The figure shows three views and two pictorial views of one solid part (mm, origin at its lowest corner). Answer the questions. A direction names the side the tool comes from. Coordinates: 2 decimals unless noted, no trailing zeros. Order: outer loops, then holes, each group sorted by start corner. A loop starts at its lowest first (then second) coordinate and runs counter-clockwise, first axis right, second up. Notation, with made-up numbers: (-15, 16) -> (29, 16) arc R16 ccw to (29, 46) -> close; hole circle Ø1 at (-6, 18.5). An arc over 180 degrees is marked (long way). Write item = value, one per line.
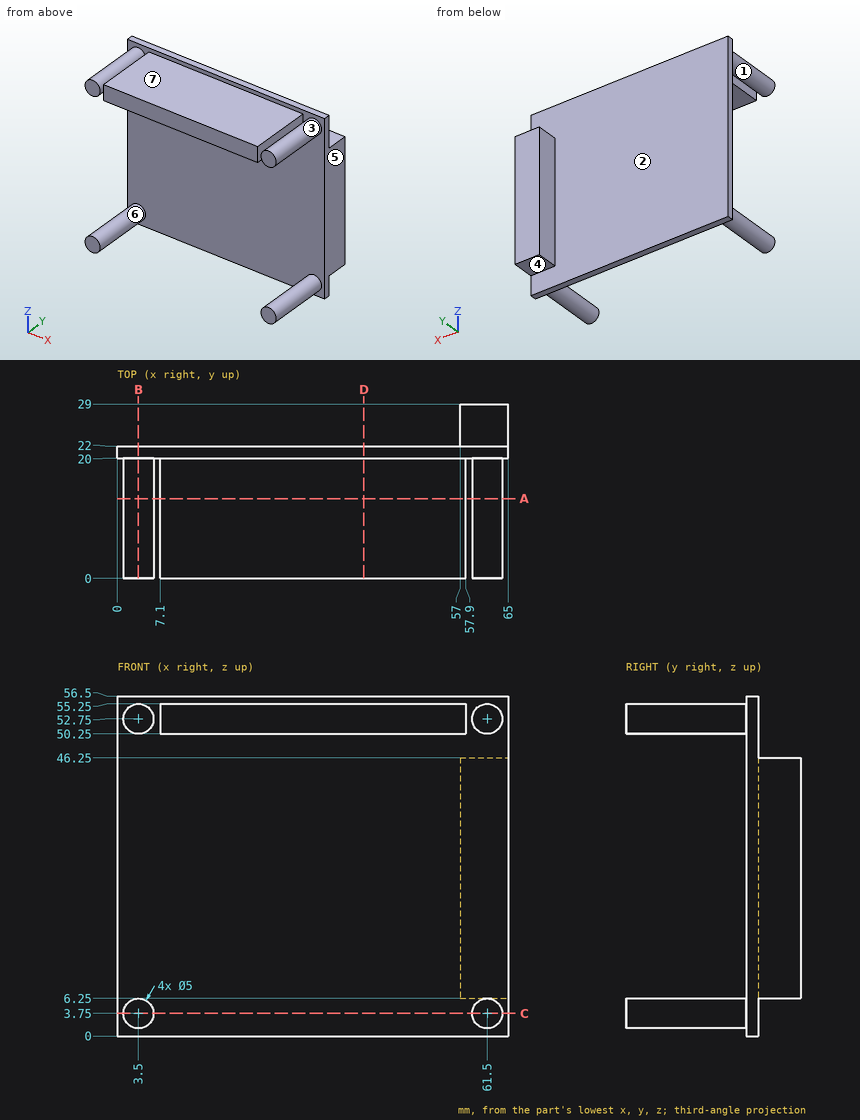
Q1. Find the intervals of material crossed by line 1 along X through (y, z) = (7, 50.5); line 2 along Z through (x, y) = (19.5, 7); line 3 along X through (y, z) = (26.75, 8.5), in increasing order.
The answers:
line_1 = 2.41 to 4.59, 7.1 to 57.9, 60.41 to 62.59
line_2 = 50.25 to 55.25
line_3 = 57 to 65
Q2. The mould has two halves that part along Z. Classify the marked faces 1, 2, 3 and 4: released by +Z, released by -Z, zero draft, split by the parting line, or undercut.
The answers:
face_1 = undercut
face_2 = zero draft
face_3 = undercut
face_4 = released by -Z
Q3. Section A-A, the plane y = 13.25 is taken. Give the vertices of the cut face in (x, z).
The answers:
outline = circle Ø5 at (3.5, 3.75); circle Ø5 at (3.5, 52.75); (7.1, 50.25) -> (57.9, 50.25) -> (57.9, 55.25) -> (7.1, 55.25) -> close; circle Ø5 at (61.5, 3.75); circle Ø5 at (61.5, 52.75)
Q4. A tool of negligible diameter and unlimited length cuts with its end or side. For the marked faces 5, 6 and 7, from which of +Z, -Z, +X, -X, +Y, -Y can it reach the whole face along a straight path? Write none if from no direction.
The answers:
face_5 = +Z, -Z, +X, +Y, -Y
face_6 = -Y
face_7 = +Z, +X, -X, -Y
Q5. Section C-C, the plane z = 3.75 is taken. Give the vertices of the cut face in (x, y).
The answers:
outline = (0, 20) -> (1, 20) -> (1, 0) -> (6, 0) -> (6, 20) -> (59, 20) -> (59, 0) -> (64, 0) -> (64, 20) -> (65, 20) -> (65, 22) -> (0, 22) -> close
Q6. Each of these flat-tipped pins is pushed along its axis until it touches: pin 1 Ø12 at (x, z) = (9, 21) entering from -Y; pin 2 Ø8 at (x, z) = (12.5, 9.5) entering from +Y; pin 3 Ø5.5 at (y, z) = (27, 17.5) entering from -X; pin 4 Ø6 at (y, z) = (4.5, 11.5) entering from +X. Where does it stop, or does it pass through?
The answers:
pin_1 = 20
pin_2 = 22
pin_3 = 57
pin_4 = through
Q7. Section D-D, the plane x = 41 is taken. Give the vertices of the cut face in (y, z).
The answers:
outline = (0, 50.25) -> (20, 50.25) -> (20, 0) -> (22, 0) -> (22, 56.5) -> (20, 56.5) -> (20, 55.25) -> (0, 55.25) -> close
Q8. Section B-B, the plane x = 3.5 is taken. Give the vertices of the cut face in (y, z).
The answers:
outline = (0, 1.25) -> (20, 1.25) -> (20, 0) -> (22, 0) -> (22, 56.5) -> (20, 56.5) -> (20, 55.25) -> (0, 55.25) -> (0, 50.25) -> (20, 50.25) -> (20, 6.25) -> (0, 6.25) -> close
